The model under review builds one solid part; all positions refer to its coordinate system, in mm. Face numbers are marked on the shaded views. A direction names the side the tool comes from. Give positions to 0.01 mm unless a question says otherwise; leave off trailing zeros. Write each loop counter-clockwise with the first axis right and the second up, starting at its lowest first coordinate (ties: lowest second). Pieces come first, ordered by that corner, then holes. Notation, with made-up numbers: (62.25, -39.5) - (71.25, -39.5) arc R29 ccw to (71.25, -2.5) - close; hole circle Ø2 at (-9, -25.75). An arc over 180 degrees is marked (long way). One line per question, with ' | ' between items. Start each with the question number.
```python
from build123d import *

# Parameters (mm, degrees)
F3_DEPTH = 1
F4_R     = 8.7131724749
F5_DEPTH = 1


with BuildPart() as f1:
    # F0 (on Top) → F1 (revolve)
    with BuildSketch(Plane.XY):
        with BuildLine():
            Line((-3.9494680241, 50.3856427968), (-11.8484050035, 50.3856427968))
            ThreePointArc((-11.8484050035, 50.3856427968), (-12.128128908, 33.9480583368), (-16.3962785155, 18.0718079209))
            Line((-16.3962785155, 18.0718079209), (-3.9494680241, 18.0718079209))
            Line((-3.9494680241, 18.0718079209), (-3.9494680241, 50.3856427968))
        make_face()
    revolve(axis=Axis((-3.9494680241, 34.2287253588, 0), (0, -1, 0)))

    # F2 (on face) → F3 (join)
    with BuildSketch(Plane.XZ.offset(-18.0718079209)):
        with BuildLine():
            ThreePointArc((20.8871186327, -2.8537629964), (21.0096452056, -1.4292189441), (21.0505319759, 0))
            ThreePointArc((21.0505319759, 0), (21.0096452056, 1.4292189441), (20.8871186327, 2.8537629964))
            Line((20.8871186327, 2.8537629964), (20.8871186327, -0.0005340841))
            Line((20.8871186327, -0.0005340841), (20.8871186327, -2.8537629964))
        make_face()
        with BuildLine():
            Line((20.8871186327, -0.0005340841), (20.8871186327, 2.8537629964))
            ThreePointArc((20.8871186327, 2.8537629964), (12.7495750458, 18.6048907696), (-3.7860546809, 24.9994659159))
            Line((-3.7860546809, 24.9994659159), (-4.1128813673, 24.9994659159))
            Line((-4.1128813673, 24.9994659159), (-4.1128813673, -0.0005340841))
            Line((-4.1128813673, -0.0005340841), (20.8871186327, -0.0005340841))
        make_face()
        with BuildLine():
            ThreePointArc((-3.7860546809, 24.9994659159), (12.7495750458, 18.6048907696), (20.8871186327, 2.8537629964))
            Line((20.8871186327, 2.8537629964), (20.8871186327, 24.9994659159))
            Line((20.8871186327, 24.9994659159), (-3.7860546809, 24.9994659159))
        make_face()
        with BuildLine():
            Line((20.8871186327, -25.0005340841), (20.8871186327, -2.8537629964))
            ThreePointArc((20.8871186327, -2.8537629964), (-5.3784203627, -24.9591284947), (-28.9494680184, -0.0005340841))
            Line((-28.9494680184, -0.0005340841), (-29.1128813673, -0.0005340841))
            Line((-29.1128813673, -0.0005340841), (-29.1128813673, -25.0005340841))
            Line((-29.1128813673, -25.0005340841), (20.8871186327, -25.0005340841))
        make_face()
        with BuildLine():
            ThreePointArc((-28.9494680184, -0.0005340841), (-5.3784203627, -24.9591284947), (20.8871186327, -2.8537629964))
            Line((20.8871186327, -2.8537629964), (20.8871186327, -0.0005340841))
            Line((20.8871186327, -0.0005340841), (-4.1128813673, -0.0005340841))
            Line((-4.1128813673, -0.0005340841), (-28.9494680184, -0.0005340841))
        make_face()
        with BuildLine():
            Line((-4.1128813673, 24.9994659159), (-3.7860546809, 24.9994659159))
            ThreePointArc((-3.7860546809, 24.9994659159), (-3.9494680241, 25), (-4.1128813673, 24.9994659159))
        make_face()
        with BuildLine():
            Line((-29.1128813673, -0.0005340841), (-28.9494680184, -0.0005340841))
            ThreePointArc((-28.9494680184, -0.0005340841), (-21.6850069981, 17.6196100213), (-4.1128813673, 24.9994659159))
            Line((-4.1128813673, 24.9994659159), (-29.1128813673, 24.9994659159))
            Line((-29.1128813673, 24.9994659159), (-29.1128813673, -0.0005340841))
        make_face()
        with BuildLine():
            ThreePointArc((-4.1128813673, 24.9994659159), (-21.6850069981, 17.6196100213), (-28.9494680184, -0.0005340841))
            Line((-28.9494680184, -0.0005340841), (-4.1128813673, -0.0005340841))
            Line((-4.1128813673, -0.0005340841), (-4.1128813673, 24.9994659159))
        make_face()
    extrude(amount=F3_DEPTH)

    # F4 (on face) → F5 (join)
    with BuildSketch(Plane(origin=(0, 50.3856427968, 0), x_dir=(-1, 0, 0), z_dir=(0, 1, 0))):
        with Locations((3.9494680241, 0)):
            Circle(F4_R)
    extrude(amount=F5_DEPTH)


solid = f1.part
```
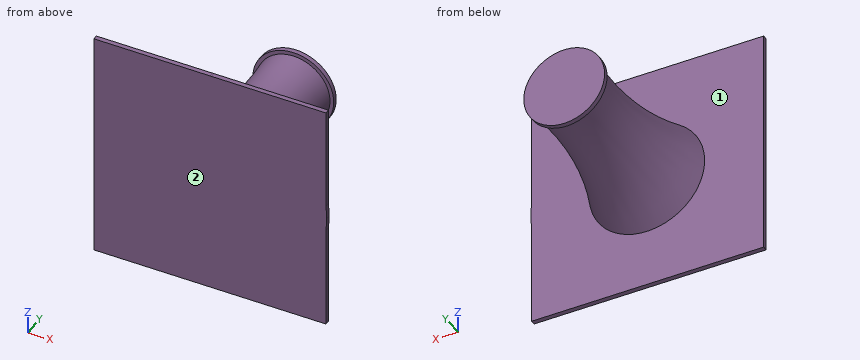
Item 1: Take a section at C-C (y = 23.5). Give the boundary of the cut face in (x, z), plus the area to 3 significant figures.
Item 2: Take a section at D-D (y = 44). Give the boundary of the cut face in (x, z), plus the area to 3 significant figures.
Item 3: Take a section at A-A (z = -21.5). Give the boundary of the cut face in (x, y), plus the area to 3 significant figures.
Item 4: For probe 1 along Y at (x, z) = (-20, -13.5); probe 2 along X at (y, z) = (20, 7.5); probe 3 along Y at (x, z) = (-14, 6), list the stretches that pass through material, from the lowest coordinate up.
Item 5: Take a section at B-B (x = -22.5). Give the boundary of the cut face in (y, z), plus the area to 3 significant figures.
Item 6: Machinability: for the marked faces 1 and 2, which of the approach directions +Z, -Z, +X, -X, +Y, -Y give a long, thin tool a straight path to every point of the face, cutting with its end or side? Answer none if there is none.
Item 7: Clearance check with flat-ended pins moving along their axes: P1, Ø5, axis at x = -0.5, y = 28, coming from the +Z side; P2, Ø4, axis at x = -8.5, z = 15.5, coming from the +Y side; P3, Ø2, axis at x = -7.5, y = 29.5, coming from the -Z side. State where each tip first meets the part, or that it passes through.
Check sheet entries:
1) outline: circle Ø21.02 at (-3.95, 0) | area: 347 mm^2
2) outline: circle Ø15.05 at (-3.95, 0) | area: 178 mm^2
3) outline: (-29.11, 17.07) - (20.89, 17.07) - (20.89, 18.07) - (-29.11, 18.07) - close | area: 50.0 mm^2
4) probe 1: y = 17.07 to 18.07 | probe 2: x = -12.93 to 5.03 | probe 3: y = 17.07 to 19.98
5) outline: (17.07, -25) - (18.07, -25) - (18.07, 25) - (17.07, 25) - close | area: 50.0 mm^2
6) face 1: +Y | face 2: +Z, -Z, +X, -X, -Y
7) P1: stops at z = 9.6 | P2: stops at y = 18.07 | P3: stops at z = -8.66
